For this review, take the finished solid that the model builds, in its own axes (mm). Face numbers are marked on the shaded views. A direction names the side the tool comes from. Round coordinates to 2 decimals unless told otherwise and drop trailing zeros. Write each loop counter-clockwise with the first axis right and the second up, starting at its lowest first coordinate (ties: lowest second). Pieces come first, ordered by that corner, then holes.
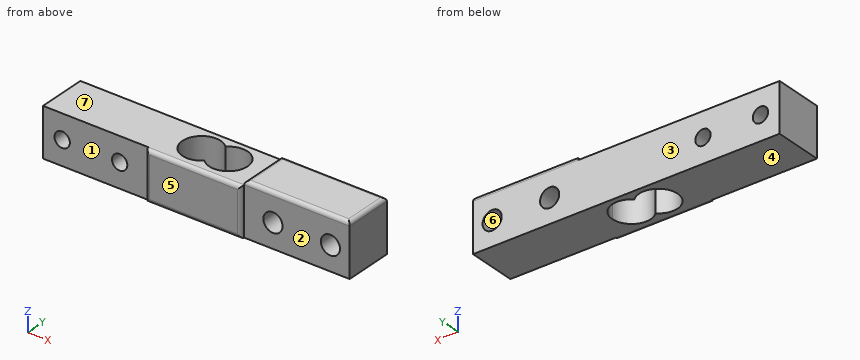
from build123d import *

# Parameters (mm, degrees)
F0_W     = 80
F0_H     = 12.7
F1_DEPTH = 6.35
F2_R     = 2
F2_R_2   = 2.5
F3_DEPTH = 12.701
F5_DEPTH = 12.701
F6_W     = 25
F6_H     = 12.7
F7_DEPTH = 1
F8_W     = 27.5
F8_H     = 12.7
F9_DEPTH = 1
F10_R    = 0.99999


# Not quite as in the source:
# - a fillet or chamfer is up to 0.001 mm smaller than in the source, because OpenCascade refuses the exact size


with BuildPart() as f1:
    # F0 (on Front) → F1 (new body, symmetric)
    with BuildSketch(Plane.XZ):
        Rectangle(F0_W, F0_H)
    extrude(amount=F1_DEPTH, both=True)

    # F2 (on face) → F3 (cut, through all)
    with BuildSketch(Plane.XZ.offset(6.35)):
        with Locations((-35, 0)):
            Circle(F2_R)
        with Locations((-20, 0)):
            Circle(F2_R)
        with Locations((35, 0)):
            Circle(F2_R_2)
        with Locations((20, 0)):
            Circle(F2_R_2)
    extrude(amount=-F3_DEPTH, mode=Mode.SUBTRACT)

    # F4 (on face) → F5 (cut, through all)
    with BuildSketch(Plane.XY.offset(6.35)):
        with BuildLine():
            ThreePointArc((0, -3.5707142143), (5.4364916731, -4.6097722286), (8.5, 0))
            ThreePointArc((8.5, 0), (5.4364916731, 4.6097722286), (0, 3.5707142143))
            ThreePointArc((0, 3.5707142143), (1.1097722286, 1.9364916731), (1.5, 0))
            ThreePointArc((1.5, 0), (1.1097722286, -1.9364916731), (0, -3.5707142143))
        make_face()
        with BuildLine():
            ThreePointArc((1.5, 0), (1.1097722286, 1.9364916731), (0, 3.5707142143))
            ThreePointArc((0, 3.5707142143), (-1.5, 0), (0, -3.5707142143))
            ThreePointArc((0, -3.5707142143), (1.1097722286, -1.9364916731), (1.5, 0))
        make_face()
        with BuildLine():
            ThreePointArc((0, -3.5707142143), (-1.5, 0), (0, 3.5707142143))
            ThreePointArc((0, 3.5707142143), (-8.5, 0), (0, -3.5707142143))
        make_face()
    extrude(amount=-F5_DEPTH, mode=Mode.SUBTRACT)

    # F6 (on face) → F7 (join)
    with BuildSketch(Plane.XZ.offset(6.35)):
        Rectangle(F6_W, F6_H)
    extrude(amount=F7_DEPTH)

    # F8 (on face) → F9 (join)
    with BuildSketch(Plane.XY.offset(6.35)):
        with Locations((26.25, 0)):
            Rectangle(F8_W, F8_H)
    extrude(amount=F9_DEPTH)

    # F10 (radius 1 in the source; OpenCascade refuses exactly that, so slightly less here)
    f10_edges = [f1.edges().sort_by_distance(p)[0] for p in [
        (12.5, 0, 7.35),
        (40, 0, 7.35),
        (0, -7.35, 6.35),
        (0, -7.35, -6.35),
        (12.5, -7.35, 0),
        (-12.5, -7.35, 0),
        (26.25, 6.35, 7.35),
        (26.25, -6.35, 7.35),
    ]]
    fillet(f10_edges, radius=F10_R)


solid = f1.part
(1) For line 1 along Z through (x, y) = (-35, 1.5); line 2 along Z through (x, y) = (35, 3); line 3 along X through (y, z) = (2, 1), list the stretches that pass through material, from the lowest coordinate up.
Geometry check:
line 1: z = -6.35 to -2, 2 to 6.35
line 2: z = -6.35 to -2.5, 2.5 to 7.35
line 3: x = -40 to -36.73, -33.27 to -21.73, -18.27 to -8.08, 8.08 to 17.71, 22.29 to 32.71, 37.29 to 40
(2) For the marked faces 1, 2 and 3, list the 3-axis set-ups (+Z, -Z, +X, -X, +Y, -Y) from which the entire face can be reached by the end or side of a thin tool; tool diameter is ignored.
Geometry check:
face 1: +Z, -Z, -X, -Y
face 2: +Z, -Z, +X, -Y
face 3: +Z, -Z, +X, -X, +Y
(3) Mouldability with a two-part tool opening along Z and no side actions: class the marked faces 4, 5, 6 and 7 as pulls with the +Z half, pulls with the -Z half, needs draft (parallel to the pull), parting line crosses it, or undercut.
Geometry check:
face 4: pulls with the -Z half
face 5: needs draft
face 6: undercut
face 7: pulls with the +Z half
(4) We need section B-B, the plane y = 2.75. State how many separate pieces and enclosed holes the cut face has, and give its area (3 significant figures).
Geometry check:
separate pieces: 2
enclosed holes: 4
area: 784 mm2
(5) For pin 1 Ø4 at (x, z) = (27.5, 1) entering from -Y; pin 2 Ø6.5 at (x, y) = (-13.5, 1.5) entering from +Z; pin 3 Ø3.5 at (x, z) = (-20, 0) entering from +Y, all flat-tipped, find the tip position at first contact; note any pin that passes through.
Geometry check:
pin 1: stops at y = -6.35
pin 2: stops at z = 6.35
pin 3: passes through
(6) We need section A-A, the plane x = 6.5. Give the boundary of the cut face in (y, z), and give its area (3 significant figures).
Geometry check:
outline: (-7.35, -5.35) arc R1 ccw to (-6.35, -6.35) - (-4, -6.35) - (-4, 6.35) - (-6.35, 6.35) arc R1 ccw to (-7.35, 5.35) - close; (4, -6.35) - (6.35, -6.35) - (6.35, 6.35) - (4, 6.35) - close
area: 72.0 mm2
